from build123d import *

# Parameters (mm, degrees)
SKETCH1_R                 = 14
EXTRUDE1_DEPTH            = 88.76
M4X0_7_TAPPED_HOLE1_D     = 3.3
M4X0_7_TAPPED_HOLE1_DEPTH = 5.029
M4X0_7_TAPPED_HOLE1_TIP   = 0.991420021
CIRPATTERN1_COUNT         = 3
CIRPATTERN1_ANGLE         = 180
SKETCH6_R                 = 11.447205948
EXTRUDE2_DEPTH            = 5
EXTRUDE3_DEPTH            = 1
EXTRUDE3_DEPTH_BACK       = 7
SKETCH7_R                 = 3.118608258


with BuildPart() as part:
    # Sketch1 → Extrude1 (new body)
    with BuildSketch(Plane(origin=(0, 0, 0), x_dir=(1, 0, 0), z_dir=(0, 1, 0))):
        with Locations(Location((0, 0, 0), (0, 0, 90))):
            Circle(SKETCH1_R)
    extrude(amount=EXTRUDE1_DEPTH)

    # M4x0.7 Tapped Hole1
    with Locations(Plane(origin=(-1.120603621, 0, -3.903834828), x_dir=(-1, 0, 0), z_dir=(0, -1, 0))):
        with Locations((-1.120603621, -3.903834828)):
            Hole(M4X0_7_TAPPED_HOLE1_D / 2, depth=M4X0_7_TAPPED_HOLE1_DEPTH)
            with Locations((0, 0, -(M4X0_7_TAPPED_HOLE1_DEPTH + M4X0_7_TAPPED_HOLE1_TIP / 2))):  # 118° drill point
                Cone(0, M4X0_7_TAPPED_HOLE1_D / 2, M4X0_7_TAPPED_HOLE1_TIP, mode=Mode.SUBTRACT)

    # Sketch4 → 8-32 Tapped Hole1 (revolve, cut)
    with BuildSketch(Plane(origin=(-14, 41, 0), x_dir=(0, 0, 1), z_dir=(0, 1, 0))):
        Polygon((0, 0), (0, 11.745806461), (1.7272, 10.708), (1.7272, 0), align=None)
    f_8_32_tapped_hole1 = revolve(axis=Axis((-20.35, 41, 0), (1, 0, 0)), mode=Mode.SUBTRACT)

    # CirPattern1: 8-32 Tapped Hole1 ×3 about axis
    cirpattern1_axis = Axis((0, 0, 0), (0, 1, 0))
    for i in range(1, CIRPATTERN1_COUNT):
        add(f_8_32_tapped_hole1.rotate(cirpattern1_axis, i * CIRPATTERN1_ANGLE / (CIRPATTERN1_COUNT - 1)), mode=Mode.SUBTRACT)

    # Sketch6 → Extrude2 (cut)
    with BuildSketch(Plane(origin=(0, 88.76, 0), x_dir=(1, 0, 0), z_dir=(0, 1, 0))):
        with Locations(Location((0, 0, 0), (0, 0, 270))):
            Circle(SKETCH6_R)
    extrude(amount=-EXTRUDE2_DEPTH, mode=Mode.SUBTRACT)

    # Sketch7 → Extrude3 (add, two sides: drawn at the far end of the back side and taken through both)
    with BuildSketch(Plane.XY.offset(-14).offset(-EXTRUDE3_DEPTH_BACK)):
        with Locations((0, 41)):
            Circle(SKETCH7_R)
    extrude(amount=EXTRUDE3_DEPTH + EXTRUDE3_DEPTH_BACK)


solid = part.part
Design review of the part built by this model. Coordinates are the model's own, in mm. A direction names the side the tool comes from. Round coordinates to 2 decimals unless told otherwise and drop trailing zeros. Write each loop counter-clockwise with the first axis right and the second up, starting at its lowest first coordinate (ties: lowest second). Pieces come first, ordered by that corner, then holes. Notation, with made-up numbers: (65.25, 40.5) - (74.25, 40.5) arc R9 ccw to (74.25, 51.5) - close; hole circle Ø6 at (-38, -8.5). An arc over 180 degrees is marked (long way). Return JSON: item names as keys, results as strings. Group by question number.
Item 1: We need section B-B on z = -7.5. Write out the cut boundary in (x, y).
Item 2: Insertion check: P1, Ø3, axis at y = 41, z = 0, coming from the -X side; P2, Ø4, axis at x = 6.5, y = 74.5, coming from the -Z side; P3, Ø6, axis at y = 77.5, z = -12, coming from the +X side. Each pin has a flat end and moves straight along its axis. Give the tip position at first contact, or say it passes through.
Item 3: For probe 1 along X at (y, z) = (86, 0); probe 2 along Y at (x, z) = (-6.75, 0); probe 3 along Z at (x, y) = (-7, 41), list the stretches that pass through material, from the lowest coordinate up. Write a range as [from, to].
Item 4: We need section A-A on x = -5.25. Write out the cut boundary in (y, z).
Item 5: Machinability: for faces 5 (the face through (-0.374, 42.686, 8.721)), 6 (the face through (-1.216, 2.55, -1.115)), 7 (the face through (0, 83.76, 0)), 8 (the face through (-8.721, 42.686, -0.374)), 9 (the face through (8.721, 42.686, 0.374)), which of the approach directions +Z, -Z, +X, -X, +Y, -Y give a long, thin tool a straight path to every point of the face, cutting with its end or side? Answer none if there is none.
Item 6: We need section C-C on x = 10.5. Write out the cut boundary in (y, z), and give its area (3 significant figures).
Item 7: The part is to be moulded in two halves that separate along Y. For faces 1 (the face through (0.138, 41.266, 2.434)), 2 (the face through (-2.1, 88.76, 11.5)), 3 (the face through (0, 41, -21)), 4 (the face through (-2.434, 41.266, 0.138)), say which applies: pulls with the +Y half, pulls with the -Y half, needs draft (parallel to the pull), parting line crosses it, or undercut.
Item 8: We need section D-D on y = 82. Write out the cut boundary in (x, z).
Model answer:
{
 "1": {"outline": "(-11.82, 0) - (11.82, 0) - (11.82, 88.76) - (8.65, 88.76) - (8.65, 83.76) - (-8.65, 83.76) - (-8.65, 88.76) - (-11.82, 88.76) - close"},
 "2": {"P1": "stops at x = -3.16", "P2": "stops at z = -13.26", "P3": "stops at x = 10.72"},
 "3": {"probe 1": "x = [-14, -11.45], [11.45, 14]", "probe 2": "y = [0, 39.27], [42.73, 83.76]", "probe 3": "z = [-12.12, -1.73], [1.73, 12.12]"},
 "4": {"outline": "(0, -12.98) - (88.76, -12.98) - (88.76, -10.17) - (83.76, -10.17) - (83.76, 10.17) - (88.76, 10.17) - (88.76, 12.98) - (0, 12.98) - close; hole circle Ø3.45 at (41, 0)"},
 "5": {"face 5": "+Z", "face 6": "-Y", "face 7": "+Y", "face 8": "-X", "face 9": "+X"},
 "6": {"outline": "(0, -9.26) - (88.76, -9.26) - (88.76, -4.56) - (83.76, -4.56) - (83.76, 4.56) - (88.76, 4.56) - (88.76, 9.26) - (0, 9.26) - close; hole circle Ø3.45 at (41, 0)", "area": "1,590 mm²"},
 "7": {"face 1": "undercut", "face 2": "pulls with the +Y half", "face 3": "needs draft", "face 4": "undercut"},
 "8": {"outline": "circle Ø28 at (0, 0)"}
}
